Could you check a few things on this drawing? It's one solid part, dimensions in mm from its lowest x, y, z. Give positions to 0.01 mm unless a question says otherwise; leave off trailing zeros. Order: outer loops, then holes, each group sorted by start corner. A loop starts at its lowest first (then second) coordinate and runs counter-clockwise, first axis right, second up. Notation, with made-up numbers: M 6,19 L 38,19 A27 cw 38,41 Z; hole C -27.5,60.25 d10. An arc over 180 degrees is marked long. Use one line per item in the form item = value. Start each with the question number.
1. I need wall thicknesses on L1, parallel to Z at x = 6, y = 5; L2, parallel to X at y = 8.5, z = 15.75; L3, parallel to Z at x = 10.5, y = 0.5. Which ranges of each line are inside material? Lowest first, please.
2. Will this pin go through, and if not, where does the flat tip stop? P1, Ø6, axis at y = 7.5, z = 23.5, coming from the +X side.
3. I want a section at C-C, the plane z = 28. List the corners of the cut face in (x, y) for me, and give its area (3 significant figures).
4. I want a section at B-B, the plane x = 3. List the corners of the cut face in (y, z) for me.
5. I want a section at A-A, the plane y = 9.25. List the corners of the cut face in (x, z) for me, and give its area (3 significant figures).
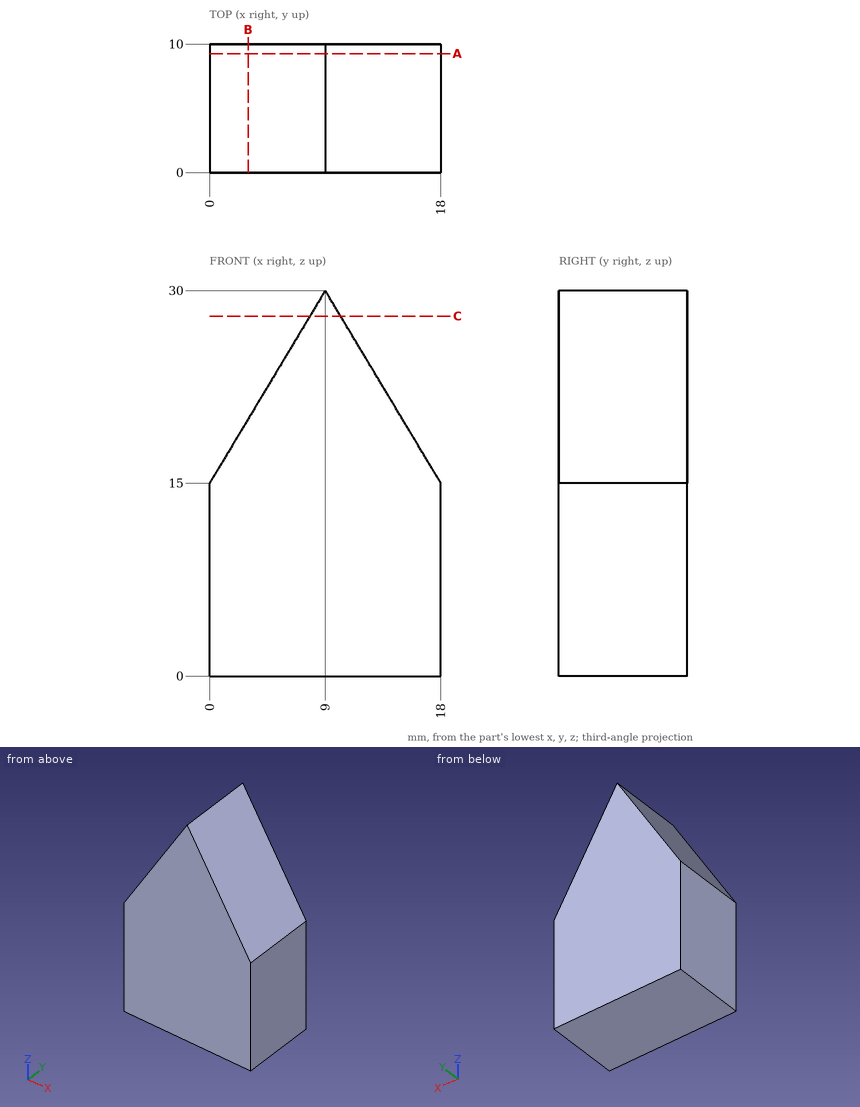
Check result:
q1.L1 = 0 to 25
q1.L2 = 0.45 to 17.55
q1.L3 = 0 to 27.5
q2.P1 = 14.7
q3.outline = M 7.8,0 L 10.2,0 L 10.2,10 L 7.8,10 Z
q3.area = 24.0 mm2
q4.outline = M 0,0 L 10,0 L 10,20 L 0,20 Z
q5.outline = M 0,0 L 18,0 L 18,15 L 9,30 L 0,15 Z
q5.area = 405 mm2
